Autodesk Inventor part; units mm, degrees
ref_plane "YZ Plane" through (0, 0, 0) normal (1, 0, 0) x (0, 1, 0)
ref_plane "XZ Plane" through (0, 0, 0) normal (0, 1, 0) x (-1, 0, 0)
ref_plane "XY Plane" through (0, 0, 0) normal (0, 0, 1) x (1, 0, 0)
sketch "Sketch1" plane through (0, 0, 0) normal (0, 1, 0) x (-1, 0, 0)
  line L0 (0, 0) -> (0, -71.12)
  line L1 (0, -71.12) -> (71.12, -71.12)
  line L2 (71.12, -71.12) -> (71.12, 0)
  line L3 (71.12, 0) -> (0, 0)
  arc A0 (71.12, -71.12) -> (71.12, 0) centre (-71.8439, -35.56) ccw
  arc A1 (0, 0) -> (0, -71.12) centre (142.9639, -35.56) ccw
  arc A2 (0, -71.12) -> (71.12, -71.12) centre (35.56, 71.8439) ccw
  arc A3 (71.12, 0) -> (0, 0) centre (35.56, -142.9639) ccw
  circle A4 centre (35.56, -35.56) radius 24.13
  dimension "d9" = 71.12
  dimension "d10" = 71.12
  dimension "d14" = 147.32
  dimension "d17" = 48.26
  dimension "d18" = 35.56
  dimension "d19" = 35.56
extrude "Extrusion1" add sketch "Sketch1" along normal blind 3.81
fillet "Fillet1" radius 3.175 4 edges at (0, 1.905, 0) (0, 1.905, -71.12) (-71.12, 1.905, 0) (-71.12, 1.905, -71.12)
sketch "Sketch2" plane through (0, 3.81, 0) normal (0, 1, 0) x (1, 0, 0)
  point P0 (0, 0)
sketch "Sketch3" plane through (0, 0, 0) normal (0, -1, 0) x (1, 0, 0)
  circle A0 centre (-35.56, -35.56) radius 24.13
  circle A1 centre (-35.56, -35.56) radius 31.75
  circle A2 centre (-35.56, -35.56) radius 24.13
  point P0 (0, 0)
  dimension "d23" = 63.5
extrude "Extrusion2" cut sketch "Sketch3" against normal blind 2.1079
sketch "Sketch4" plane through (0, 0, 0) normal (0, -1, 0) x (1, 0, 0)
  circle A0 centre (-35.56, -35.56) radius 24.13
  circle A1 centre (-35.56, -35.56) radius 31.75
  circle A2 centre (-60.96, -10.16) radius 1.905
  arc A3 (-1.9053, 0.4605) -> (-69.2147, 0.4605) centre (-35.56, -142.9639) ccw construction
  line L0 (-35.56, 4.3561) -> (-35.56, -75.4761) construction
  arc A4 (-69.2147, -71.5805) -> (-1.9053, -71.5805) centre (-35.56, 71.8439) ccw construction
  arc A5 (-71.5805, -1.9053) -> (-71.5805, -69.2147) centre (71.8439, -35.56) ccw construction
  line L1 (-75.4761, -35.56) -> (4.3561, -35.56) construction
  arc A6 (0.4605, -69.2147) -> (0.4605, -1.9053) centre (-142.9639, -35.56) ccw construction
  line L2 (-75.4761, -35.56) -> (-75.4761, 1.4435) construction
  circle A7 centre (-10.16, -10.16) radius 1.905
  line L3 (4.3561, -35.56) -> (4.3561, 1.4435) construction
  circle A8 centre (-60.96, -60.96) radius 1.905
  circle A9 centre (-10.16, -60.96) radius 1.905
  point P0 (0, 0)
  dimension "d26" = 3.81
  dimension "d34" = 25.4
  dimension "d35" = 25.4
  dimension "d36" = 14.5161
  dimension "d37" = 14.5162
  dimension "d38" = 50.8
  dimension "d39" = 50.8
extrude "Extrusion3" cut sketch "Sketch4" against normal blind 25.4 contours A2 | A7 | A8 | A9
sketch "Sketch6" plane through (0, 0, 0) normal (0, -1, 0) x (1, 0, 0)
  point P0 (0, 0)
sketch "Sketch8" plane through (0, 3.81, 0) normal (0, 1, 0) x (1, 0, 0)
  circle A0 centre (-35.56, 35.56) radius 24.13
  circle A1 centre (-35.56, 35.56) radius 24.13 construction
  line L0 (-35.56, 59.69) -> (-35.56, 64.77) construction
  line L1 (-35.56, 11.43) -> (-35.56, 6.35) construction
  line L2 (-11.43, 35.56) -> (-6.35, 35.56) construction
  arc A2 (-35.56, 6.35) -> (-35.56, 64.77) centre (-35.56, 35.56) ccw
  line L3 (-35.56, 64.77) -> (-35.56, 6.35)
  point P0 (0, 0)
  dimension "d44" = 5.08
  dimension "d45" = 5.08
  dimension "d46" = 5.08
extrude "Extrusion5" add sketch "Sketch8" along normal blind 3.556 contours A0 L3 | A0 L3 A2 picked at (-27.7183, 37.3498)
fillet "Fillet2" radius 3.048 1 edges at (-6.35, 3.81, -35.56)
properties part number "_3DPrint"
Build history of the part. All positions in model axes, mm. A direction names the side the tool comes from. Give positions to 0.01 mm unless a question says otherwise; leave off trailing zeros. Loops run counter-clockwise (first coordinate to the right, second up) from the corner with the lowest first, then second, coordinate; pieces in that order, holes last.
Item 1: Pull direction X, two halves, no side cores. Call faces 1 (the face through (-61.21, 1.88, -59.07)), 2 (the face through (4.355, 1.878, -36.035)), 3 (the face through (-16.41, 2.95, -20.88)), 4 (the face through (-53, 3.81, -17)): released by +X, released by -X, zero draft, split by the parting line, or undercut.
Answers follow:
face 1: undercut
face 2: released by +X
face 3: undercut
face 4: zero draft
Item 2: Flat gauge pins, fed straight in: pin 1 (4 mm diameter, centred on y = 1, z = -16.5, fed in from -X) (3 decimals); pin 2 (1.5 mm diameter, centred on y = 4, z = -54, fed in from +X); pin 3 (3 mm diameter, centred on x = -57, z = -21.5, fed in from -Y). Where does each tip first touch, or does it go through?
Answers follow:
pin 1: stops at x = -74.485
pin 2: stops at x = 3.29
pin 3: stops at y = 2.11
Item 3: Slice it at C-C, the plane x = -60.96. List the corners of the cut face in (y, z) (3 decimals).
Answers follow:
outline: (0, -73.27) - (3.81, -73.27) - (3.81, -62.865) - (0, -62.865) - close; (0, -59.055) - (3.81, -59.055) - (3.81, -12.065) - (0, -12.065) - (0, -16.51) - (2.108, -16.51) - (2.108, -54.61) - (0, -54.61) - close; (0, -8.255) - (3.81, -8.255) - (3.81, 2.15) - (0, 2.15) - close
Item 4: Drill centre lines: line 1 (Z direction, x = -60.96, y = 2.15) (3 decimals); line 2 (Y direction, x = -1.5, z = -15.5); line 3 (Z direction, x = -60.96, y = 0.8) (3 decimals). Where is each one in solid material? Low to high.
Answers follow:
line 1: z = -73.27 to -62.865, -59.055 to -12.065, -8.255 to 2.15
line 2: y = 0 to 3.81
line 3: z = -73.27 to -62.865, -59.055 to -54.61, -16.51 to -12.065, -8.255 to 2.15
Item 5: Slice it at A-A, the plane z = -35.56. List the corners of the cut face in (x, y).
Answers follow:
outline: (-75.48, 0) - (-67.31, 0) - (-67.31, 2.11) - (-59.69, 2.11) - (-59.69, 3.81) - (-75.48, 3.81) - close; (-35.56, 3.81) - (-11.43, 3.81) - (-11.43, 2.11) - (-3.81, 2.11) - (-3.81, 0) - (4.36, 0) - (4.36, 3.81) - (-3.3, 3.81) arc R3.05 cw to (-6.35, 6.86) - (-6.35, 7.37) - (-35.56, 7.37) - close
Item 6: Slice it at D-D, the plane z = -60.96. Give the number of separate pieces and of enclosed holes in the cut face, and give its area (3 significant figures).
Answers follow:
separate pieces: 3
enclosed holes: 0
area: 233 mm2
Item 7: Which spindle directions (+Z, -Z, +X, -X, +Y, -Y) get a long thin tool onto all of the face, cutting with end or side? Do faces 5 (the face through (-29, 2.108, -12)), 6 (the face through (-6.357, 7.108, -36.202)), 7 (the face through (-35.56, 6, -36)). Say none if no direction does.
Answers follow:
face 5: -Y
face 6: +X, +Y
face 7: +Z, -Z, -X, +Y
Item 8: Slice it at B-B, the plane x = -43. List the corners of the cut face in (y, z), and give its area (3 significant figures).
Answers follow:
outline: (0, -75.29) - (3.81, -75.29) - (3.81, -58.51) - (2.11, -58.51) - (2.11, -66.43) - (0, -66.43) - close; (0, -4.69) - (2.11, -4.69) - (2.11, -12.61) - (3.81, -12.61) - (3.81, 4.17) - (0, 4.17) - close
area: 94.5 mm2
